Geometry check sheet. Reference: the model listing, model coordinates, mm. Face numbers are marked on the shaded views. A direction names the side the tool comes from. Coordinates: 2 decimals unless noted, no trailing zeros. Write each loop counter-clockwise with the first axis right and the second up, starting at its lowest first coordinate (ties: lowest second). Pieces come first, ordered by that corner, then holes.
from build123d import *
from build123d.topology import SkipClean

# Parameters (mm, degrees)
SKETCH_1_R          = 4.9
EXTRUDE_1_DEPTH     = 25.3
SKETCH_1_R_2        = 3.15
EXTRUDE_1_2_DEPTH   = 25.3
SKETCH_1_R_3        = 8
SKETCH_1_R_4        = 5.25
EXTRUDE_1_3_DEPTH   = 25.3
EXTRUDE_START       = 5
SKETCH_2_R          = 3.15
EXTRUDE_2_DEPTH     = 5
SKETCH_3_W          = 101.378011207
SKETCH_3_H          = 57.539128355
CUT_EXTRUDE_1_DEPTH = 15.3
CUT_EXTRUDE_2_DEPTH = 100.289108802
FILLET_1_R          = 3
SKETCH_5_R          = 5.25
CUT_EXTRUDE_3_DEPTH = 100.289108802
EXTRUDE_3_DEPTH     = 2


with BuildPart() as part:
    # Sketch 1 → Extrude 1 (new body)
    with BuildSketch(Plane(origin=(0, 0, 0), x_dir=(1, 0, 0), z_dir=(0, 1, 0))):
        with Locations(Location((44.713737374, -77.299234731, 0), (0, 0, 270))):
            Circle(SKETCH_1_R)
    extrude(amount=EXTRUDE_1_DEPTH)



with BuildPart() as body_2:
    # Sketch 1 → Extrude 1 2 (new body)
    with BuildSketch(Plane(origin=(0, 0, 0), x_dir=(1, 0, 0), z_dir=(0, 1, 0))):
        with Locations(Location((-29.536262626, -77.299234731, 0), (0, 0, 270))):
            Circle(SKETCH_1_R_2)
    extrude(amount=EXTRUDE_1_2_DEPTH)


with BuildPart() as body_3:
    # Sketch 1 → Extrude 1 3 (new body)
    with BuildSketch(Plane(origin=(0, 0, 0), x_dir=(1, 0, 0), z_dir=(0, 1, 0))):
        with Locations(Location((0, 0, 0), (0, 0, 270))):
            Circle(SKETCH_1_R_3)
        with Locations(Location((0, 0, 0), (0, 0, 270))):
            Circle(SKETCH_1_R_4, mode=Mode.SUBTRACT)
    extrude(amount=EXTRUDE_1_3_DEPTH)


with BuildPart() as part_1:
    with SkipClean():  # the faces are left unmerged after this step: merging them gives an invalid solid
        add(part.part)

        add(body_2.part)  # Extrude 2 merges body 2

        add(body_3.part)  # Extrude 2 merges body 3
        # Sketch 2 → Extrude 2 (add)
        with BuildSketch(Plane.XZ.offset(EXTRUDE_START)):
            with BuildLine():
                Line((44.482889179, 82.193793865), (-29.536262626, 80.449234731))
                ThreePointArc((-29.536262626, 80.449234731), (-27.308876266, 79.526621092), (-26.386262626, 77.299234731))
                ThreePointArc((-26.386262626, 77.299234731), (-29.049069338, 74.187138541), (-32.535559579, 76.336572905))
                Line((-32.535559579, 76.336572905), (-7.999251158, -0.109457316))
                ThreePointArc((-7.999251158, -0.109457316), (-2.503564236, -7.598168603), (6.367372109, -4.843198574))
                Line((6.367372109, -4.843198574), (49.035233225, 74.989543494))
                ThreePointArc((49.035233225, 74.989543494), (48.916563034, 79.818412468), (44.713737374, 82.199234731))
                Line((44.713737374, 82.199234731), (44.482889179, 82.193793865))
            make_face()
            with Locations(Location((-29.536262626, 77.299234731, 0), (0, 0, 90))):
                Circle(SKETCH_2_R)
        extrude(amount=-EXTRUDE_2_DEPTH)

    # Sketch 3 → Cut-Extrude 1 (cut)
    with SkipClean():  # the faces are left unmerged after this step: merging them gives an invalid solid
        with BuildSketch(Plane(origin=(0, 25.3, 0), x_dir=(1, 0, 0), z_dir=(0, 1, 0))):
            with Locations((10.685297464, -78.742909524)):
                Rectangle(SKETCH_3_W, SKETCH_3_H)
        extrude(amount=-CUT_EXTRUDE_1_DEPTH, mode=Mode.SUBTRACT)

    # Sketch 4 → Cut-Extrude 2 (cut, through all)
    with SkipClean():  # the faces are left unmerged after this step: merging them gives an invalid solid
        with BuildSketch(Plane(origin=(0, 0, 0), x_dir=(1, 0, 0), z_dir=(0, 1, 0))):
            Polygon((36.330866648, -73.997214663), (-21.007135718, -72.645813934), (0.235470884, -6.461736097), align=None)
        extrude(amount=-CUT_EXTRUDE_2_DEPTH, mode=Mode.SUBTRACT)

    # Fillet 1
    # the kernel refuses this fillet: 3 mm, written as the material it adds along each edge
    with BuildSketch(Plane(origin=(0.235470884, 0, 6.461736097), x_dir=(0.4713655585699632, 0, 0.8819379287648461), z_dir=(0, -1, 0))) as fillet_1_piece_1:
        with BuildLine():
            CenterArc((FILLET_1_R * 2.36056709959, FILLET_1_R), FILLET_1_R, 135.917656387, 134.082343613)
            Line((FILLET_1_R * 1.642226382, FILLET_1_R * 1.69569146426), (0, 0))
            Line((0, 0), (FILLET_1_R * 2.36056709959, 0))
        make_face()
    extrude(amount=5)
    with BuildSketch(Plane(origin=(36.330866648, 0, 73.997214663), x_dir=(-0.4713655585699637, 0, -0.8819379287648459), z_dir=(0, -1, 0))) as fillet_1_piece_2:
        with BuildLine():
            CenterArc((FILLET_1_R * 1.71380475401, -FILLET_1_R), FILLET_1_R, 90, 119.473130073)
            Line((FILLET_1_R * 0.843218222551, -FILLET_1_R * 1.49201533639), (0, 0))
            Line((0, 0), (FILLET_1_R * 1.71380475401, 0))
        make_face()
    extrude(amount=5)
    with BuildSketch(Plane(origin=(-21.007135718, 0, 72.645813934), x_dir=(0.999722366227584, 0, 0.023562480012096054), z_dir=(0, -1, 0))) as fillet_1_piece_3:
        with BuildLine():
            CenterArc((FILLET_1_R * 1.33781102221, -FILLET_1_R), FILLET_1_R, 90, 106.444526314)
            Line((FILLET_1_R * 0.37871675356, -FILLET_1_R * 1.28308688393), (0, 0))
            Line((0, 0), (FILLET_1_R * 1.33781102221, 0))
        make_face()
    extrude(amount=5)

    # Sketch 5 → Cut-Extrude 3 (cut, through all)
    with BuildSketch(Plane(origin=(0, 0, 0), x_dir=(1, 0, 0), z_dir=(0, 1, 0))):
        with Locations(Location((0, 0, 0), (0, 0, 90))):
            Circle(SKETCH_5_R)
    extrude(amount=-CUT_EXTRUDE_3_DEPTH, mode=Mode.SUBTRACT)

    # Sketch 6 → Extrude 3 (add)
    with BuildSketch(Plane(origin=(0, 0, 0), x_dir=(1, 0, 0), z_dir=(0, 1, 0))):
        Polygon((-0.026686724, -73.14030263), (-0.026686724, -81.144746621), (14.973313276, -81.498281975), (14.973313276, -73.493837984), align=None)
    extrude(amount=EXTRUDE_3_DEPTH)


solid = part_1.part
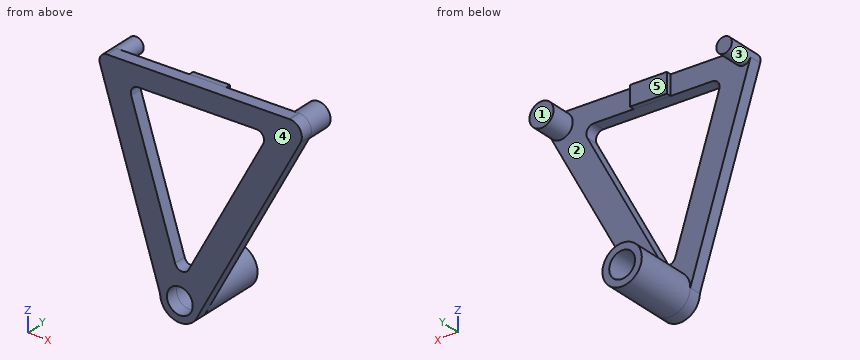
1. Draft check along X on the marked faces 3, 4 and 5. Enter one of: released by +X, released by -X, zero draft, split by the parting line, or undercut.
Computed values:
face 3: undercut
face 4: zero draft
face 5: undercut
2. Access from +Z, -Z, +X, -X, +Y, -Y to the whole of each face (thin tool, end or side, straight path). Record for the marked faces 1 and 2.
Computed values:
face 1: +Z, -Z, +X, -X, +Y
face 2: +Y
3. Sectioned sample at B-B, the plane y = 18.5. Record the boundary of the cut face in (x, z).
Computed values:
outline: circle Ø16 at (0, 0); hole circle Ø10.5 at (0, 0)
4. Sectioned sample at A-A, the plane z = 50. Record the boundary of the cut face in (x, y).
Computed values:
outline: (-24.08, -5) - (-13.74, -5) - (-13.74, 0) - (-24.08, 0) - close; (23.51, -5) - (35.68, -5) - (35.68, 0) - (23.51, 0) - close
5. Thickness scan on line 1 along X through (y, z) = (6.25, 0); line 2 along Y through (x, z) = (-3, 73.5); line 3 along X through (y, z) = (-1.2, 0). Record the ranges inside material, lowest first.
Computed values:
line 1: x = -8 to -5.25, 5.25 to 8
line 2: y = -5 to 0
line 3: x = -8.03 to -5.25, 5.25 to 8.96
6. Sectioned sample at C-C, the plane x = 36. Record the boundary of the cut face in (y, z).
Computed values:
outline: (-5, 50.6) - (0, 50.6) - (0, 81.99) - (-5, 81.99) - close
7. Gauge pin test, flat ends, axial feed: pin 1 Ø8 at (x, z) = (12, 15.5) entering from +Y; pin 2 Ø1 at (y, z) = (1.5, 79) entering from -X; pin 3 Ø2 at (x, y) = (9.5, 0) entering from +Z; pin 4 Ø8.5 at (x, z) = (0, 0) entering from -Y. Record the tip position at first contact, or that the pin passes through.
Computed values:
pin 1: stops at y = 0
pin 2: stops at x = -32.45
pin 3: stops at z = 81.39
pin 4: passes through
